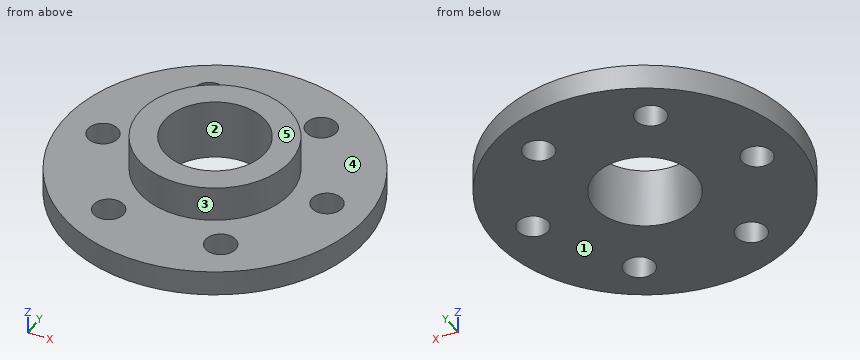
```python
from build123d import *

# Parameters (mm, degrees)
CYLINDER003_R     = 3
CYLINDER003_DEPTH = 10
ARRAY_COUNT       = 6
CYLINDER002_R     = 10
CYLINDER002_DEPTH = 30
CYLINDER001_R     = 15
CYLINDER001_DEPTH = 12
CYLINDER_R        = 30
CYLINDER_DEPTH    = 5


with BuildPart() as array:
    # Cylinder003 → Cylinder003 (new body)
    with BuildSketch(Plane(origin=(22, 0, -1), x_dir=(1, 0, 0), z_dir=(0, 0, 1))):
        Circle(CYLINDER003_R)
    extrude(amount=CYLINDER003_DEPTH)

    # Array: Array ×6 about axis
    array_axis = Axis((0, 0, 0), (0, 0, 1))


with BuildPart() as array_1:
    add(array.part)
    for i in range(1, ARRAY_COUNT):
        add(array.part.rotate(array_axis, i * 360 / ARRAY_COUNT))


with BuildPart() as tub_interior:
    # Cylinder002 → Cylinder002 (new body)
    with BuildSketch(Plane.XY.offset(-1)):
        Circle(CYLINDER002_R)
    extrude(amount=CYLINDER002_DEPTH)


with BuildPart() as tub_exterior:
    # Cylinder001 → Cylinder001 (new body)
    with BuildSketch(Plane.XY):
        Circle(CYLINDER001_R)
    extrude(amount=CYLINDER001_DEPTH)


with BuildPart() as cut001:
    # Cylinder → Cylinder (new body)
    with BuildSketch(Plane.XY):
        Circle(CYLINDER_R)
    extrude(amount=CYLINDER_DEPTH)

    # Fusion: union tub_exterior
    add(tub_exterior.part)

    # Cut: cut tub_interior
    add(tub_interior.part, mode=Mode.SUBTRACT)

    # Cut001: cut Array
    add(array_1.part, mode=Mode.SUBTRACT)


solid = cut001.part
```
Source: CAD feature listing. Evaluate the final solid. Frame: model axes, mm. Face numbers are marked on the shaded views. A direction names the side the tool comes from. Coordinates: 2 decimals unless noted, no trailing zeros. Write each loop counter-clockwise with the first axis right and the second up, starting at its lowest first coordinate (ties: lowest second). Pieces come first, ordered by that corner, then holes. Notation, with made-up numbers: (57.5, -10.75) -> (74.5, -10.75) arc R30 cw to (74.5, 27.25) -> close; hole circle Ø10 at (17.25, 51.5). An arc over 180 degrees is marked (long way). Return JSON: item names as keys, results as strings. Group by question number.
1) Section query C-C, the plane x = -11. Return loops of the section in (y, z).
2) Set-up query: the marked faces 4 and 5. Return all of +Z, -Z, +X, -X, +Y, -Y with unobstructed straight access to the full face (end or side cutting, diameter ignored); none if empty.
3) Section query A-A, the plane y = 0. Return loops of the section in (x, z).
4) Section query D-D, the plane y = -18. Return loops of the section in (x, z).
5) Section query B-B, the plane x = 0.5. Return loops of the section in (y, z), plus the area to 3 significant figures.
6) Contact query for flat-ended pins moving along their axis: P1, Ø3.5, axis at x = 11, y = -19.05, coming from the -Z side; P2, Ø5, axis at x = -9, z = 2, coming from the +Y side; P3, Ø6, axis at x = 6, z = 9, coming from the +Y side. Output: stop coordinate, or through.
7) Mould query, pull axis Y, two halves, no side actions, for the marked faces 1, 2 and 3. Classes: +Y half, -Y half, draft (parallel to the pull), parting line (faces both ways), or undercut.
8) Ray query, line 1 along X through (y, z) = (0, 6); line 2 along X through (y, z) = (-19, 1.25); line 3 along X through (y, z) = (-19.5, 2). Return the intervals inside material, ascending.
From the geometry:
{
 "1": {"outline": "(-27.91, 0) -> (-22.05, 0) -> (-22.05, 5) -> (-27.91, 5) -> close; (-16.05, 0) -> (16.05, 0) -> (16.05, 5) -> (10.2, 5) -> (10.2, 12) -> (-10.2, 12) -> (-10.2, 5) -> (-16.05, 5) -> close; (22.05, 0) -> (27.91, 0) -> (27.91, 5) -> (22.05, 5) -> close"},
 "2": {"face 4": "+Z", "face 5": "+Z, +X, -X, +Y, -Y"},
 "3": {"outline": "(-30, 0) -> (-25, 0) -> (-25, 5) -> (-30, 5) -> close; (-19, 0) -> (-10, 0) -> (-10, 12) -> (-15, 12) -> (-15, 5) -> (-19, 5) -> close; (10, 0) -> (19, 0) -> (19, 5) -> (15, 5) -> (15, 12) -> (10, 12) -> close; (25, 0) -> (30, 0) -> (30, 5) -> (25, 5) -> close"},
 "4": {"outline": "(-24, 0) -> (-13.81, 0) -> (-13.81, 5) -> (-24, 5) -> close; (-8.19, 0) -> (8.19, 0) -> (8.19, 5) -> (-8.19, 5) -> close; (13.81, 0) -> (24, 0) -> (24, 5) -> (13.81, 5) -> close"},
 "5": {"outline": "(-30, 0) -> (-9.99, 0) -> (-9.99, 12) -> (-14.99, 12) -> (-14.99, 5) -> (-30, 5) -> close; (9.99, 0) -> (30, 0) -> (30, 5) -> (14.99, 5) -> (14.99, 12) -> (9.99, 12) -> close", "area": "270 mm²"},
 "6": {"P1": "through", "P2": "y = 29.29", "P3": "y = 14.7"},
 "7": {"face 1": "draft", "face 2": "undercut", "face 3": "parting line"},
 "8": {"line 1": "-15 to -10, 10 to 15", "line 2": "-23.22 to -14, -8 to 8, 14 to 23.22", "line 3": "-22.8 to -13.97, -8.03 to 8.03, 13.97 to 22.8"}
}
